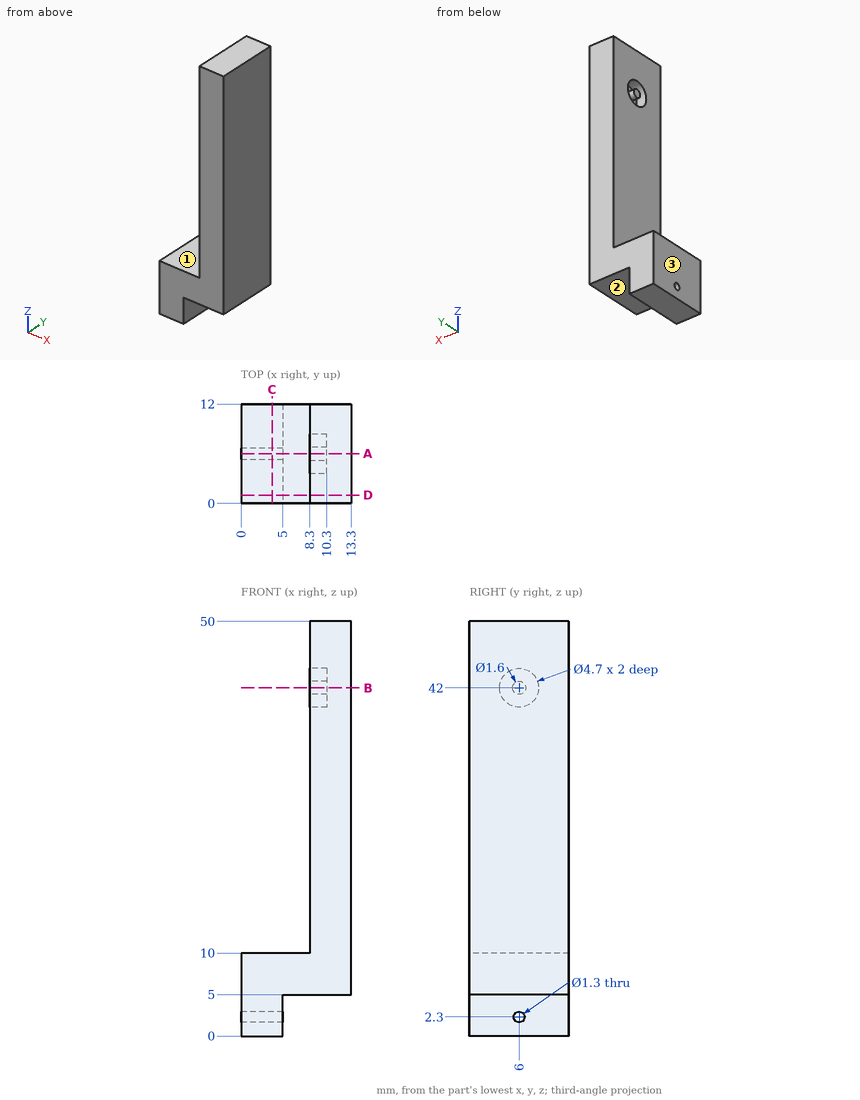
Geometry check sheet. Reference: drawing and pictorial views, mm from the part's lowest x, y, z. A direction names the side the tool comes from. Round coordinates to 2 decimals unless told otherwise and drop trailing zeros. Write each loop counter-clockwise with the first axis right and the second up, starting at its lowest first coordinate (ties: lowest second). Pieces come first, ordered by that corner, then holes.
1. Section check B-B on z = 42. Enter the section's corners in (x, y), plus the area to 3 significant figures.
2. Gauge pin test, flat ends, axial feed: P1, Ø2, axis at y = 3.5, z = 35, coming from the -X side; P2, Ø4, axis at y = 5.5, z = 2, coming from the +X side; P3, Ø4, axis at x = 5, z = 27, coming from the -Y side; P4, Ø4, axis at x = 4.5, y = 3.5, coming from the +Z side. Record the tip position at first contact, or that the pin passes through.
3. Scan lines: L1, parallel to Z at x = 8.7, y = 6; L2, parallel to Z at x = 1.95, y = 6; L3, parallel to X at y = 2, z = 21. Record each from-to range of solid material in increasing order.
4. Section check C-C on x = 3.75. Enter the section's corners in (y, z).
5. Section check D-D on y = 1. Enter the section's corners in (x, z).
6. Access from +Z, -Z, +X, -X, +Y, -Y to the whole of each face (thin tool, end or side, straight path). Record for the marked faces 1, 2 and 3.
7. Section check A-A on y = 6. Enter the section's corners in (x, z), plus the area to 3 significant figures.
Answer:
1. outline: (8.3, 0) - (13.3, 0) - (13.3, 12) - (8.3, 12) - (8.3, 8.35) - (10.3, 8.35) - (10.3, 6.8) - (8.3, 6.8) - (8.3, 5.2) - (10.3, 5.2) - (10.3, 3.65) - (8.3, 3.65) - close
1. area: 53.8 mm2
2. P1: stops at x = 8.3
2. P2: stops at x = 5
2. P3: passes through
2. P4: stops at z = 10
3. L1: z = 5 to 39.65, 41.2 to 42.8, 44.35 to 50
3. L2: z = 0 to 1.65, 2.95 to 10
3. L3: x = 8.3 to 13.3
4. outline: (0, 0) - (12, 0) - (12, 10) - (0, 10) - close; hole circle Ø1.3 at (6, 2.3)
5. outline: (0, 0) - (5, 0) - (5, 5) - (13.3, 5) - (13.3, 50) - (8.3, 50) - (8.3, 10) - (0, 10) - close
6. face 1: +Z, -X, +Y, -Y
6. face 2: -Z, +X, +Y, -Y
6. face 3: +Z, -Z, -X, +Y, -Y
7. outline: (0, 0) - (5, 0) - (5, 1.65) - (0, 1.65) - close; (0, 2.95) - (5, 2.95) - (5, 5) - (13.3, 5) - (13.3, 50) - (8.3, 50) - (8.3, 44.35) - (10.3, 44.35) - (10.3, 42.8) - (8.3, 42.8) - (8.3, 41.2) - (10.3, 41.2) - (10.3, 39.65) - (8.3, 39.65) - (8.3, 10) - (0, 10) - close
7. area: 279 mm2
